```python
from build123d import *

# Parameters (mm, degrees)
SKETCH1_W                             = 100
SKETCH1_H                             = 100
SKETCH1_R                             = 32
BOSS_EXTRUDE3_DEPTH                   = 6.35
M4_CLEARANCE_HOLE2_D                  = 4.5
M4_CLEARANCE_HOLE2_CSINK_D            = 4.55
M4_CLEARANCE_HOLE2_CSINK_ANGLE        = 90
TAP_DRILL_FOR_M3X0_5_TAP2_D           = 2.5
TAP_DRILL_FOR_M3X0_5_TAP2_DEPTH       = 9.248924226
TAP_DRILL_FOR_M3X0_5_TAP2_CSINK_D     = 2.55
TAP_DRILL_FOR_M3X0_5_TAP2_CSINK_ANGLE = 90
TAP_DRILL_FOR_M3X0_5_TAP2_TIP         = 0.751075774
TAP_DRILL_FOR_M3X0_5_TAP3_D           = 2.5
TAP_DRILL_FOR_M3X0_5_TAP3_DEPTH       = 9.248924226
TAP_DRILL_FOR_M3X0_5_TAP3_CSINK_D     = 2.55
TAP_DRILL_FOR_M3X0_5_TAP3_CSINK_ANGLE = 90
TAP_DRILL_FOR_M3X0_5_TAP3_TIP         = 0.751075774


with BuildPart() as part:
    # Sketch1 → Boss-Extrude3 (new body)
    with BuildSketch(Plane(origin=(0, 0, 0), x_dir=(1, 0, 0), z_dir=(0, 1, 0))):
        Rectangle(SKETCH1_W, SKETCH1_H)
        with Locations(Location((0, 0, 0), (0, 0, 270))):
            Circle(SKETCH1_R, mode=Mode.SUBTRACT)
    extrude(amount=BOSS_EXTRUDE3_DEPTH)

    # M4 Clearance Hole2 (through all)
    with Locations(Plane(origin=(0, 0, 0), x_dir=(-1, 0, 0), z_dir=(0, -1, 0))):
        with Locations((-9.188076101, 34.290366833), (25.102290732, 25.102290732), (34.290366833, -9.188076101), (9.188076101, -34.290366833), (-25.102290732, -25.102290732), (-34.290366833, 9.188076101)):
            CounterSinkHole(M4_CLEARANCE_HOLE2_D / 2, M4_CLEARANCE_HOLE2_CSINK_D / 2, counter_sink_angle=M4_CLEARANCE_HOLE2_CSINK_ANGLE)

    # Tap Drill for M3x0.5 Tap2
    with Locations(Plane.XY.offset(50)):
        with Locations((-35, 3.175), (35, 3.175)):
            CounterSinkHole(TAP_DRILL_FOR_M3X0_5_TAP2_D / 2, TAP_DRILL_FOR_M3X0_5_TAP2_CSINK_D / 2, depth=TAP_DRILL_FOR_M3X0_5_TAP2_DEPTH, counter_sink_angle=TAP_DRILL_FOR_M3X0_5_TAP2_CSINK_ANGLE)
            with Locations((0, 0, -(TAP_DRILL_FOR_M3X0_5_TAP2_DEPTH + TAP_DRILL_FOR_M3X0_5_TAP2_TIP / 2))):  # 118° drill point
                Cone(0, TAP_DRILL_FOR_M3X0_5_TAP2_D / 2, TAP_DRILL_FOR_M3X0_5_TAP2_TIP, mode=Mode.SUBTRACT)

    # Tap Drill for M3x0.5 Tap3
    with Locations(Plane(origin=(0, 0, -50), x_dir=(-1, 0, 0), z_dir=(0, 0, -1))):
        with Locations((-35, 3.175), (35, 3.175)):
            CounterSinkHole(TAP_DRILL_FOR_M3X0_5_TAP3_D / 2, TAP_DRILL_FOR_M3X0_5_TAP3_CSINK_D / 2, depth=TAP_DRILL_FOR_M3X0_5_TAP3_DEPTH, counter_sink_angle=TAP_DRILL_FOR_M3X0_5_TAP3_CSINK_ANGLE)
            with Locations((0, 0, -(TAP_DRILL_FOR_M3X0_5_TAP3_DEPTH + TAP_DRILL_FOR_M3X0_5_TAP3_TIP / 2))):  # 118° drill point
                Cone(0, TAP_DRILL_FOR_M3X0_5_TAP3_D / 2, TAP_DRILL_FOR_M3X0_5_TAP3_TIP, mode=Mode.SUBTRACT)


solid = part.part
```
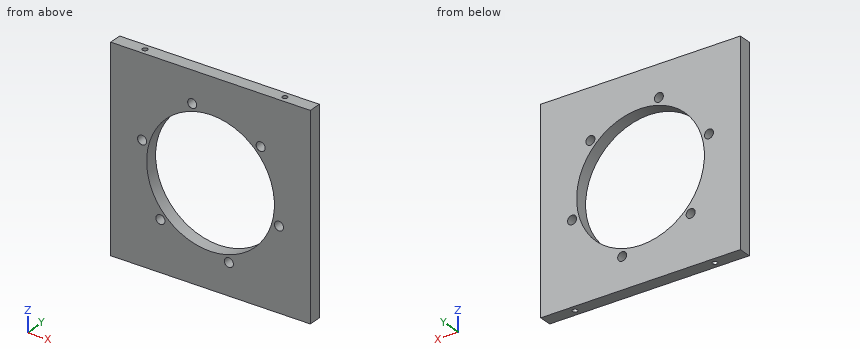
CAD build for the part. Positions are in the model's coordinates, mm. Round coordinates to 2 decimals unless told otherwise and drop trailing zeros. Order: outer loops, then holes, each group sorted by start corner. A loop starts at its lowest first (then second) coordinate and runs counter-clockwise, first axis right, second up.
Q1. Slice it at A-A (x = 0). Write the cut outline in (y, z), and give its area (3 significant figures).
Q2. Slice it at B-B (z = 0). Write the cut outline in (x, y).
Q3. Drop flat-ended pins along their axis: pin 1 (1.5 mm diameter, centred on x = -35, y = 3.175, fed in from -Z); pin 2 (2 mm diameter, centred on x = 35, y = 3.175, fed in from -Z). Give the stop position or say it passes through.
Q4. Wall check: L1, parallel to Z at x = 11, y = 4; L2, parallel to X at y = 3, z = -23.5; L3, parallel to Y at x = 35, z = 42.75 (3 decimals). Give the ranges that are in metal, low to high.
Results below:
1. outline: (0, -50) - (6.35, -50) - (6.35, -32) - (0, -32) - close; (0, 32) - (6.35, 32) - (6.35, 50) - (0, 50) - close
1. area: 229 mm2
2. outline: (-50, 0) - (-32, 0) - (-32, 6.35) - (-50, 6.35) - close; (32, 0) - (50, 0) - (50, 6.35) - (32, 6.35) - close
3. pin 1: stops at z = -40.45
3. pin 2: stops at z = -40.6
4. L1: z = -50 to -35.62, -32.96 to -30.05, 30.05 to 50
4. L2: x = -50 to -26.68, -23.52 to -21.72, 21.72 to 50
4. L3: y = 0 to 1.925, 4.425 to 6.35
